```python
from build123d import *

# Parameters (mm, degrees)
F0_W          = 10
F0_H          = 10
F1_DEPTH      = 25
F2_W          = 20
F2_H          = 20
F3_DEPTH      = 25
F4_W          = 10
F4_H          = 10
F5_DEPTH      = 5
F5_DEPTH_BACK = 15
F6_W          = 10
F6_H          = 10
F7_DEPTH      = 5
F7_DEPTH_BACK = 15


with BuildPart() as f1:
    # F0 (on Front) → F1 (new body)
    with BuildSketch(Plane.XZ):
        Rectangle(F0_W, F0_H)
    extrude(amount=F1_DEPTH)

    # F2 (on face) → F3 (join)
    with BuildSketch(Plane.XZ.offset(25)):
        Rectangle(F2_W, F2_H)
    extrude(amount=F3_DEPTH)

    # F4 (on face) → F5 (join, two sides)
    with BuildSketch(Plane.XY.offset(5)) as f5_sk:
        with Locations((0, -10)):
            Rectangle(F4_W, F4_H)
    extrude(amount=F5_DEPTH)
    extrude(f5_sk.sketch, amount=-F5_DEPTH_BACK)

    # F6 (on face) → F7 (join, two sides)
    with BuildSketch(Plane(origin=(-5, 0, 0), x_dir=(0, -1, 0), z_dir=(-1, 0, 0))) as f7_sk:
        with Locations((10, 0)):
            Rectangle(F6_W, F6_H)
    extrude(amount=F7_DEPTH)
    extrude(f7_sk.sketch, amount=-F7_DEPTH_BACK)


solid = f1.part
```
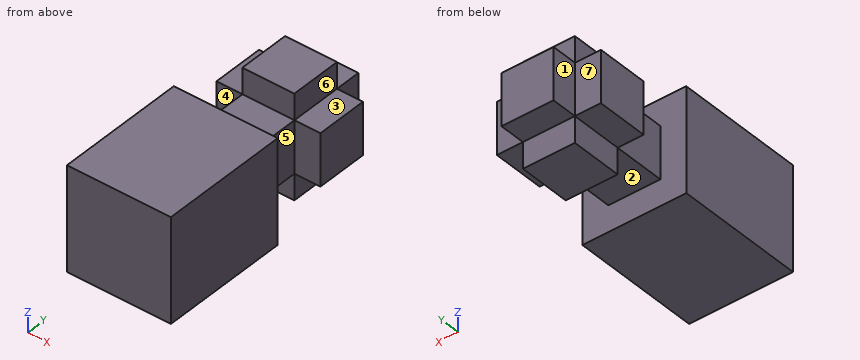
Can you work these out from the model? Positions are in its coordinate system, mm. Face numbers are marked on the shaded views. A direction names the side the tool comes from. Round coordinates to 2 decimals unless told otherwise and drop trailing zeros. Loops run counter-clockwise (first coordinate to the right, second up) from the corner with the lowest first, then second, coordinate; pieces in that order, holes last. Notation, with made-up numbers: M 89,-22 L 119,-22 A21 ccw 119,0 Z; hole C -24,34.25 d7. An arc over 180 degrees is marked long. Answer as a JSON object with one key per item and string values. Group by question number.
Q1. Imagine slicing it at B-B, the plane z = -6.5. Please give me the cut outline in (x, y).
Q2. Imagine slicing it at C-C, the plane x = -0.75. Please give me the cut outline in (y, z), then the cut area to 3 significant figures.
Q3. Imagine slicing it at A-A, the plane x = 6.25. Please give me the cut outline in (y, z).
Q4. Will these pins go through, and if not, where does the flat tip stop? pin 1 (2.5 mm diameter, centred on x = -7, y = -8.5, fed in from +Z); pin 2 (2 mm diameter, centred on y = -21.5, z = 1.5, fed in from +X); pin 3 (1.5 mm diameter, centred on x = 0.5, z = -7, fed in from +Y).
Q5. Imagine slicing it at D-D, the plane y = -14. Please give me the cut outline in (x, z).
Q6. We'd pull the mould along Y, two halves only. Please class the marked faces 4, 5, 6 and 7: +Y half, -Y half, draft (parallel to the pull), parting line (faces both ways), or undercut.
Q7. On a 3-axis mill with a long thin cutter (end or side, diameter ignored), from which of +Z, -Z, +X, -X, +Y, -Y can I reach the whole of each face in a straight line? I mean the marked faces 1, 2 and 3. Say none if no direction works.
Q8. Please list where these lines run through material, in increasing order: L1, parallel to Y at x = 7.5, z = -1.75; L2, parallel to X at y = -12.5, z = 5.25.
Findings:
{
 "1": {"outline": "M -10,-50 L 10,-50 L 10,-25 L -10,-25 Z; M -5,-15 L 5,-15 L 5,-5 L -5,-5 Z"},
 "2": {"outline": "M -50,-10 L -25,-10 L -25,-5 L -15,-5 L -15,-10 L -5,-10 L -5,-5 L 0,-5 L 0,5 L -5,5 L -5,10 L -15,10 L -15,5 L -25,5 L -25,10 L -50,10 Z", "area": "850 mm2"},
 "3": {"outline": "M -50,-10 L -25,-10 L -25,10 L -50,10 Z; M -15,-5 L -5,-5 L -5,5 L -15,5 Z"},
 "4": {"pin 1": "stops at z = 5", "pin 2": "stops at x = 5", "pin 3": "stops at y = -5"},
 "5": {"outline": "M -10,-5 L -5,-5 L -5,-10 L 5,-10 L 5,-5 L 10,-5 L 10,5 L 5,5 L 5,10 L -5,10 L -5,5 L -10,5 Z"},
 "6": {"face 4": "undercut", "face 5": "undercut", "face 6": "draft", "face 7": "+Y half"},
 "7": {"face 1": "+Z, -Z, -X, +Y", "face 2": "-Z, +X, -X", "face 3": "+Z, +X, +Y"},
 "8": {"L1": "y = -50 to -25, -15 to -5", "L2": "x = -5 to 5"}
}
